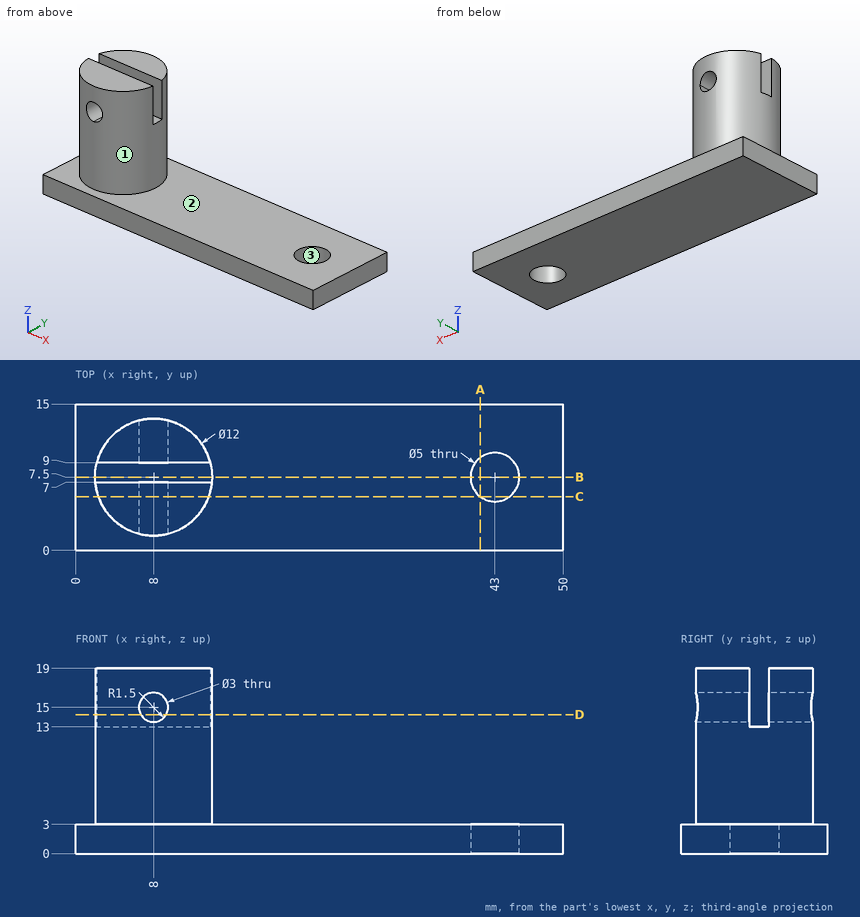
Here's the drawing with two shaded views (mm, measured from the low corner). I have some questions. Give positions to 0.01 mm unless a question says otherwise; leave off trailing zeros. Order: outer loops, then holes, each group sorted by start corner. A loop starts at its lowest first (then second) coordinate and runs counter-clockwise, first axis right, second up. Notation, with made-up numbers: (-10, 42) -> (-6, 42) arc R26 ccw to (-6, 76) -> close; hole circle Ø10 at (29.5, 6.5). An arc over 180 degrees is marked (long way). One line per item, written item: value. Start each with the question number.
1. Will these pins go through, and if not, where does the flat tip stop? pin 1 Ø6.5 at (x, y) = (43, 7.5) entering from +Z; pin 2 Ø1.8 at (x, z) = (8, 15) entering from -Y; pin 3 Ø1.5 at (y, z) = (8.5, 8.5) entering from -X; pin 4 Ø1.6 at (x, y) = (9, 8) entering from +Z.
2. I need wall thicknesses on probe 1 along Y at (x, z) = (43, 1.6); probe 2 along Z at (x, y) = (8, 12); probe 3 along Z at (x, y) = (4.5, 7.75). Which ranges of each line are inside material? Lowest first, please. Write a range as from..to.
3. Imagine slicing it at C-C, the plane y = 5.5. List the corners of the cut face in (x, z) for me, plus the area to 3 significant figures.
4. We'd pull the mould along Y, two halves only. Please class the marked faces 1, 2 and 3: released by +Y, released by -Y, zero draft, split by the parting line, or undercut.
5. Imagine slicing it at D-D, the plane z = 14.25. List the corners of the cut face in (x, y) for me, plus the area to 3 significant figures.
6. Imagine slicing it at A-A, the plane x = 41.5. List the corners of the cut face in (y, z) for me.
7. Imagine slicing it at B-B, the plane y = 7.5. List the corners of the cut face in (x, z) for me.
Values follow:
1. pin 1: stops at z = 3
1. pin 2: passes through
1. pin 3: stops at x = 2.01
1. pin 4: stops at z = 13
2. probe 1: y = 0..5, 10..15
2. probe 2: z = 0..13.5, 16.5..19
2. probe 3: z = 0..13
3. outline: (0, 0) -> (41.5, 0) -> (41.5, 3) -> (13.66, 3) -> (13.66, 19) -> (2.34, 19) -> (2.34, 3) -> (0, 3) -> close; (44.5, 0) -> (50, 0) -> (50, 3) -> (44.5, 3) -> close; hole circle Ø3 at (8, 15)
3. area: 315 mm2
4. face 1: split by the parting line
4. face 2: zero draft
4. face 3: undercut
5. outline: (2.02, 7) arc R6 ccw to (6.7, 1.64) -> (6.7, 7) -> close; (2.19, 9) -> (6.7, 9) -> (6.7, 13.36) arc R6 ccw to start; (9.3, 1.64) arc R6 ccw to (13.98, 7) -> (9.3, 7) -> close; (9.3, 9) -> (13.81, 9) arc R6 ccw to (9.3, 13.36) -> close
5. area: 63.6 mm2
6. outline: (0, 0) -> (5.5, 0) -> (5.5, 3) -> (0, 3) -> close; (9.5, 0) -> (15, 0) -> (15, 3) -> (9.5, 3) -> close
7. outline: (0, 0) -> (40.5, 0) -> (40.5, 3) -> (14, 3) -> (14, 13) -> (2, 13) -> (2, 3) -> (0, 3) -> close; (45.5, 0) -> (50, 0) -> (50, 3) -> (45.5, 3) -> close
